Build history of the part. All positions in model axes, mm. A direction names the side the tool comes from. Round coordinates to 2 decimals unless told otherwise and drop trailing zeros. Write each loop counter-clockwise with the first axis right and the second up, starting at its lowest first coordinate (ties: lowest second). Pieces come first, ordered by that corner, then holes. Notation, with made-up numbers: (47.5, 4) - (64.5, 4) arc R21 cw to (64.5, 25) - close; hole circle Ø3 at (26, 53). An arc over 180 degrees is marked (long way). Answer as a JSON object with one key per item and string values. Group by question number.
Item 1: Probe line 1 (X direction, y = -15, z = -53.5); line 2 (Y direction, x = -313, z = -90.5); line 3 (Y direction, x = -310, z = -45). List the from-to ranges inside material, lowest first. Write a range as from..to.
Item 2: Slice it at C-C, the plane x = -327. List the corners of the cut face in (y, z).
Item 3: Slice it at B-B, the plane y = -30.5. List the corners of the cut face in (x, z), then the cut area to 3 significant figures.
Item 4: Which spindle directions (+Z, -Z, +X, -X, +Y, -Y) get a long thin tool onto all of the face, cutting with end or side? Do faces 1 (the flat face through (-371, 88.9, 2)), 2 (the flat face through (-360.946, 22, 2)). Say none if no direction does.
Item 5: Slice it at A-A, the plane z = -11. List the corners of the cut face in (x, y) (3 decimals).
Item 6: Flat gauge pins, fed straight in: pin 1 (12 mm diameter, centred on y = -27, z = 49.5, fed in from +X); pin 2 (3 mm diameter, centred on x = -346.5, z = -50.5, fed in from +Y); pin 3 (4 mm diameter, centred on x = -327.5, z = -30.5, fed in from +Y). Where does each tip first touch, or does it go through?
from build123d import *

# Parameters (mm, degrees)
SKETCH1_W           = 215.9
SKETCH1_H           = 279.4
BOSS_EXTRUDE1_DEPTH = 63.5
CUT_EXTRUDE2_DEPTH  = 216.9


with BuildPart() as part:
    # Sketch1 → Boss-Extrude1 (new body, symmetric)
    with BuildSketch(Plane(origin=(-316.495998982, -92.239904424, -225.371199256), x_dir=(0, 0, -1), z_dir=(1, 0, 0))):
        with Locations((-225.371199256, 92.239904424)):
            Rectangle(SKETCH1_W, SKETCH1_H)
    extrude(amount=BOSS_EXTRUDE1_DEPTH, both=True)

    # Sketch2 → Cut-Extrude2 (cut, through all)
    with BuildSketch(Plane.XY.offset(107.95)):
        with BuildLine():
            Line((-272.045998982, -139.7), (-252.995998982, -139.7))
            Line((-252.995998982, -139.7), (-252.995998982, 139.7))
            Line((-252.995998982, 139.7), (-379.995998982, 139.7))
            Line((-379.995998982, 139.7), (-379.995998982, 88.9))
            Line((-379.995998982, 88.9), (-360.945998982, 88.9))
            Line((-360.945998982, 88.9), (-360.945998982, -47.625))
            ThreePointArc((-360.945998982, -47.625), (-334.90779183, -110.486792847), (-272.045998982, -136.525))
            Line((-272.045998982, -136.525), (-272.045998982, -139.7))
        make_face()
    extrude(amount=-CUT_EXTRUDE2_DEPTH, mode=Mode.SUBTRACT)


solid = part.part
Geometry says:
{
 "1": {"line 1": "x = -380..-360.95", "line 2": "y = -139.7..-126.53", "line 3": "y = -139.7..-128.02"},
 "2": {"outline": "(-139.7, -107.95) - (-117.51, -107.95) - (-117.51, 107.95) - (-139.7, 107.95) - close"},
 "3": {"outline": "(-380, -107.95) - (-360.95, -107.95) - (-360.95, 107.95) - (-380, 107.95) - close", "area": "4,110 mm^2"},
 "4": {"face 1": "+Z, -Z, +X, -X, +Y", "face 2": "+Z, -Z, +X, +Y"},
 "5": {"outline": "(-379.996, -139.7) - (-272.046, -139.7) - (-272.046, -136.525) arc R88.9 cw to (-360.946, -47.625) - (-360.946, 88.9) - (-379.996, 88.9) - close"},
 "6": {"pin 1": "stops at x = -360.95", "pin 2": "stops at y = -93.82", "pin 3": "stops at y = -115.46"}
}
